```python
from build123d import *

# Parameters (mm, degrees)
SKETCH_1_W          = 900
SKETCH_1_H          = 918
EXTRUDE_1_DEPTH     = 1.5
SKETCH_2_W          = 900
SKETCH_2_H          = 918
SKETCH_2_W_2        = 897
SKETCH_2_H_2        = 915
EXTRUDE_2_DEPTH     = 15
SKETCH_3_W          = 900
SKETCH_3_H          = 918
SKETCH_3_W_2        = 870
SKETCH_3_H_2        = 898
EXTRUDE_3_DEPTH     = 1.5
SKETCH_6_R          = 3
CUT_EXTRUDE_1_DEPTH = 19
FILLET_1_R          = 1


with BuildPart() as part:
    # 草图1 → 凸台-拉伸1 (new body)
    with BuildSketch(Plane.XY):
        Rectangle(SKETCH_1_W, SKETCH_1_H)
    extrude(amount=EXTRUDE_1_DEPTH)

    # 草图2 → 凸台-拉伸2 (add)
    with BuildSketch(Plane(origin=(0, 0, 0), x_dir=(-1, 0, 0), z_dir=(0, 0, -1))):
        Rectangle(SKETCH_2_W, SKETCH_2_H)
        Rectangle(SKETCH_2_W_2, SKETCH_2_H_2, mode=Mode.SUBTRACT)
    extrude(amount=EXTRUDE_2_DEPTH)

    # 草图3 → 凸台-拉伸3 (add)
    with BuildSketch(Plane(origin=(0, 0, -15), x_dir=(-1, 0, 0), z_dir=(0, 0, -1))):
        Rectangle(SKETCH_3_W, SKETCH_3_H)
        Rectangle(SKETCH_3_W_2, SKETCH_3_H_2, mode=Mode.SUBTRACT)
    extrude(amount=EXTRUDE_3_DEPTH)

    # 草图6 → 切除-拉伸1 (cut, through all)
    with BuildSketch(Plane.XY.offset(1.5)):
        with Locations((-421, -430)):
            Circle(SKETCH_6_R)
        with Locations((421, -430)):
            Circle(SKETCH_6_R)
    extrude(amount=-CUT_EXTRUDE_1_DEPTH, mode=Mode.SUBTRACT)

    # 圆角1
    fillet_1_edges = [part.edges().sort_by_distance(p)[0] for p in [
        (450, 0, 1.5),
        (0, 459, 1.5),
        (-450, 0, -16.5),
        (0, 459, -16.5),
        (450, 0, -16.5),
        (0, -459, -16.5),
        (-450, 0, 1.5),
        (0, -459, 1.5),
        (-450, 459, -7.5),
        (450, 459, -7.5),
        (450, -459, -7.5),
        (-450, -459, -7.5),
    ]]
    fillet(fillet_1_edges, radius=FILLET_1_R)


solid = part.part
```
Can you work these out from the model? Positions are in its coordinate system, mm. Round coordinates to 2 decimals unless told otherwise and drop trailing zeros. Loops run counter-clockwise (first coordinate to the right, second up) from the corner with the lowest first, then second, coordinate; pieces in that order, holes last. Notation, with made-up numbers: (74.5, 61.5) -> (78.5, 61.5) arc R32 cw to (78.5, 93.5) -> close; hole circle Ø7 at (-10.75, 26.25). An arc over 180 degrees is marked (long way). One line per item, written item: value. Start each with the question number.
1. If we section it at A-A, the plane z = -9.5: Write out the boundary of the cut face in (x, y), then the cut area to 3 significant figures.
2. If I drill on probe 1 along X at (y, z) = (-430, 1.15); probe 2 along Y at (x, z) = (-305, -8.25); probe 3 along X at (y, z) = (150.5, -9), over which ranges is the centre line in solid material (lowest first)?
3. If we section it at B-B, the plane y = -370: Write out the boundary of the cut face in (x, z).
4. For pin 1 (2 mm diameter, centred on x = 358.5, y = 361.5, fed in from -Z), with a flat end and sliding along its axis, tell me the tip position at first contact or that it passes through.
5. If we section it at C-C, the plane x = -361: Write out the boundary of the cut face in (y, z).
6. If we mould it in two halves opening along Y, with no side actions, what happens to faces 1 (the flat face through (-6, 6, 1.5)), 2 (the flat face through (-6, 6, 0))? For each: pulls with the +Y half, pulls with the -Y half, needs draft (parallel to the pull), parting line crosses it, or undercut.
Calculated:
1. outline: (-450, -458) arc R1 ccw to (-449, -459) -> (449, -459) arc R1 ccw to (450, -458) -> (450, 458) arc R1 ccw to (449, 459) -> (-449, 459) arc R1 ccw to (-450, 458) -> close; hole (-448.5, -457.5) -> (448.5, -457.5) -> (448.5, 457.5) -> (-448.5, 457.5) -> close
1. area: 5,440 mm²
2. probe 1: x = -449.76 to -424, -418 to 418, 424 to 449.76
2. probe 2: y = -459 to -457.5, 457.5 to 459
2. probe 3: x = -450 to -448.5, 448.5 to 450
3. outline: (-450, -15.5) arc R1 ccw to (-449, -16.5) -> (-435, -16.5) -> (-435, -15) -> (-448.5, -15) -> (-448.5, 0) -> (448.5, 0) -> (448.5, -15) -> (435, -15) -> (435, -16.5) -> (449, -16.5) arc R1 ccw to (450, -15.5) -> (450, 0.5) arc R1 ccw to (449, 1.5) -> (-449, 1.5) arc R1 ccw to (-450, 0.5) -> close
4. pin 1: stops at z = 0
5. outline: (-459, -15.5) arc R1 ccw to (-458, -16.5) -> (-449, -16.5) -> (-449, -15) -> (-457.5, -15) -> (-457.5, 0) -> (457.5, 0) -> (457.5, -15) -> (449, -15) -> (449, -16.5) -> (458, -16.5) arc R1 ccw to (459, -15.5) -> (459, 0.5) arc R1 ccw to (458, 1.5) -> (-458, 1.5) arc R1 ccw to (-459, 0.5) -> close
6. face 1: needs draft
6. face 2: undercut
